Here's how the part is built. I have some questions about the finished solid (model axes, mm). Face numbers are marked on the shaded views. Give positions to 0.01 mm unless a question says otherwise; leave off trailing zeros. Loops run counter-clockwise (first coordinate to the right, second up) from the corner with the lowest first, then second, coordinate; pieces in that order, holes last. Notation, with made-up numbers: (6.25, 18) - (50.25, 18) arc R16 cw to (50.25, 22) - close; hole circle Ø4 at (6, -15). An arc over 180 degrees is marked (long way). Return JSON: item names as keys, results as strings. Group by question number.
(1) If we section it at B-B (x = -5): Please give me the cut outline in (y, z).
(2) For P1, Ø6, axis at x = -5, z = 35, coming from the -Y side; P2, Ø1, axis at x = -7.5, y = 0, coming from the -Z side; P3, Ø7, axis at x = -5, z = 25, coming from the +Y side; P4, Ø2, axis at x = -4, z = 19.5, coming from the +Y side, each with a flat end and sliding along its axis, tell me the tip position at first contact or that it passes through.
(3) If we mould it in two halves opening along X, with no side actions, what happens to the marked faces 1, 2 and 3? For each: released by +X, released by -X, zero draft, split by the parting line, or undercut.
(4) I need wall thicknesses on probe 1 along X at (y, z) = (-2, 35); probe 2 along Z at (x, y) = (5, -2.5); probe 3 along Z at (x, y) = (-6, 1.75). Which ranges of each line are inside material? Lowest first, please. Write a range as [from, to].
(5) If we section it at A-A (y = -1.5): State how many separate pieces and enclosed holes the cut face has, then the cut area to 3 significant figures.
(6) If we section it at C-C (y = 4.25): Please give me the cut outline in (x, z).
(7) If we section it at D-D (z = 35): Please give me the cut outline in (x, y).
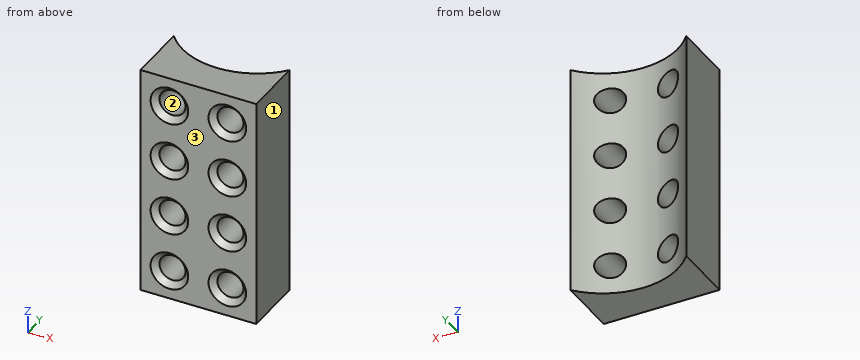
```python
from build123d import *

# Parameters (mm, degrees)
BOSS_EXTRUDE1_DEPTH = 40
SKETCH2_R           = 2.25
CUT_EXTRUDE1_DEPTH  = 43.595167487
CHAMFER1_SIZE       = 1


with BuildPart() as part:
    # Sketch1 → Boss-Extrude1 (new body)
    with BuildSketch(Plane.XY):
        with BuildLine():
            Line((-10, -5.346688069), (10, -5.346688069))
            Line((10, -5.346688069), (10, 5.346688069))
            ThreePointArc((10, 5.346688069), (0, 0.653311931), (-10, 5.346688069))
            Line((-10, 5.346688069), (-10, -5.346688069))
        make_face()
    extrude(amount=BOSS_EXTRUDE1_DEPTH)

    # Sketch2 → Cut-Extrude1 (cut, through all)
    with BuildSketch(Plane.XZ.offset(5.346688069)):
        with Locations(Location((5, 5, 0), (0, 0, 270))):
            Circle(SKETCH2_R)
        with Locations(Location((-5, 5, 0), (0, 0, 270))):
            Circle(SKETCH2_R)
        with Locations(Location((-5, 15, 0), (0, 0, 270))):
            Circle(SKETCH2_R)
        with Locations(Location((5, 15, 0), (0, 0, 270))):
            Circle(SKETCH2_R)
        with Locations(Location((-5, 25, 0), (0, 0, 270))):
            Circle(SKETCH2_R)
        with Locations(Location((5, 25, 0), (0, 0, 270))):
            Circle(SKETCH2_R)
        with Locations(Location((-5, 35, 0), (0, 0, 270))):
            Circle(SKETCH2_R)
        with Locations(Location((5, 35, 0), (0, 0, 270))):
            Circle(SKETCH2_R)
    extrude(amount=-CUT_EXTRUDE1_DEPTH, mode=Mode.SUBTRACT)

    # Chamfer1
    chamfer1_edges = [part.edges().sort_by_distance(p)[0] for p in [
        (5, -5.346688069, 27.25),
        (-5, -5.346688069, 17.25),
        (5, -5.346688069, 17.25),
        (-5, -5.346688069, 7.25),
        (-5, -5.346688069, 37.25),
        (5, -5.346688069, 37.25),
        (-5, -5.346688069, 27.25),
        (5, -5.346688069, 7.25),
    ]]
    chamfer(chamfer1_edges, length=CHAMFER1_SIZE)


solid = part.part
```
Values:
{
 "1": {"outline": "(-5.35, 0) - (1.65, 0) - (1.65, 2.75) - (-4.35, 2.75) - (-5.35, 1.75) - close; (-5.35, 8.25) - (-4.35, 7.25) - (1.65, 7.25) - (1.65, 12.75) - (-4.35, 12.75) - (-5.35, 11.75) - close; (-5.35, 18.25) - (-4.35, 17.25) - (1.65, 17.25) - (1.65, 22.75) - (-4.35, 22.75) - (-5.35, 21.75) - close; (-5.35, 28.25) - (-4.35, 27.25) - (1.65, 27.25) - (1.65, 32.75) - (-4.35, 32.75) - (-5.35, 31.75) - close; (-5.35, 38.25) - (-4.35, 37.25) - (1.65, 37.25) - (1.65, 40) - (-5.35, 40) - close"},
 "2": {"P1": "y = -5.1", "P2": "z = 0", "P3": "y = 3.82", "P4": "y = 1.65"},
 "3": {"face 1": "released by +X", "face 2": "undercut", "face 3": "zero draft"},
 "4": {"probe 1": "[-10, -7.25], [-2.75, 2.75], [7.25, 10]", "probe 2": "[0, 2.75], [7.25, 12.75], [17.25, 22.75], [27.25, 32.75], [37.25, 40]", "probe 3": "[0, 2.98], [7.02, 12.98], [17.02, 22.98], [27.02, 32.98], [37.02, 40]"},
 "5": {"separate pieces": "1", "enclosed holes": "8", "area": "673 mm2"},
 "6": {"outline": "(-10, 0) - (-8.98, 0) - (-8.98, 40) - (-10, 40) - close; (8.98, 0) - (10, 0) - (10, 40) - (8.98, 40) - close"},
 "7": {"outline": "(-10, -5.35) - (-8.25, -5.35) - (-7.25, -4.35) - (-7.25, 2.86) arc R13 cw to (-10, 5.35) - close; (-2.75, -4.35) - (-1.75, -5.35) - (1.75, -5.35) - (2.75, -4.35) - (2.75, 0.95) arc R13 cw to (-2.75, 0.95) - close; (7.25, -4.35) - (8.25, -5.35) - (10, -5.35) - (10, 5.35) arc R13 cw to (7.25, 2.86) - close"}
}
